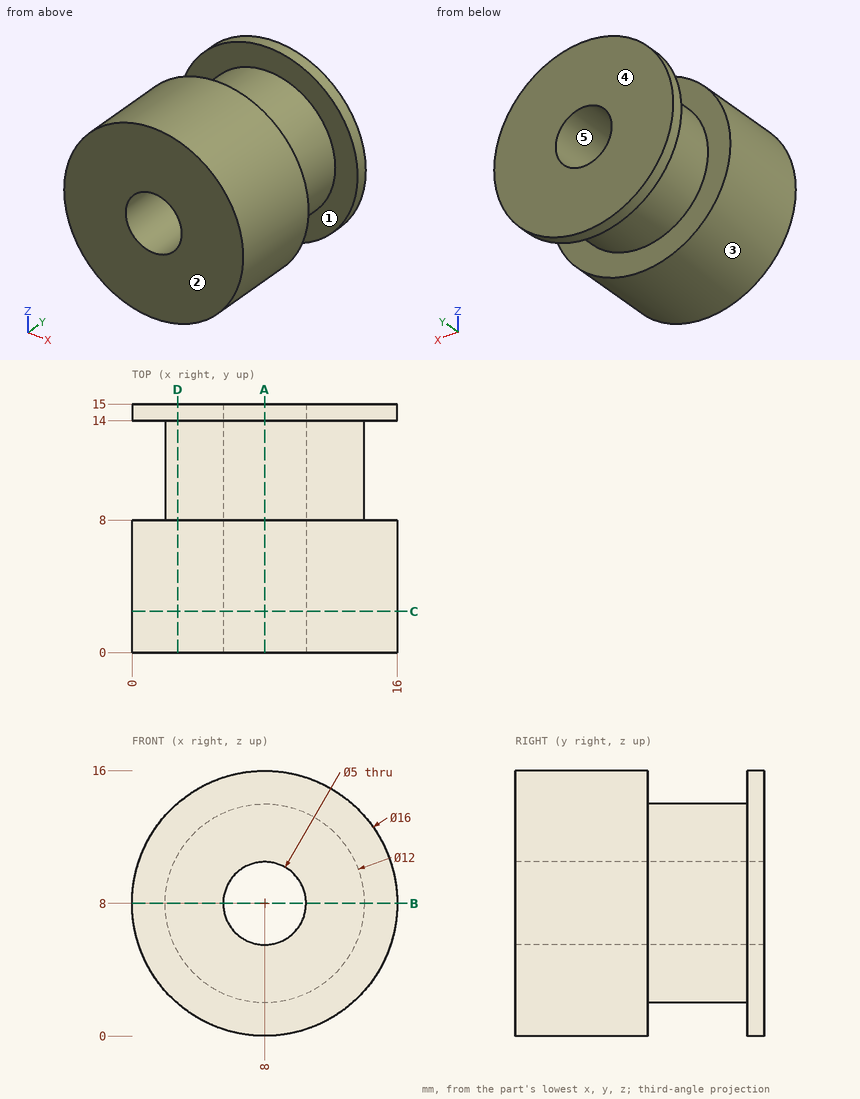
Verification items for this drawing (mm, ordinates from the low corner). A direction names the side the tool comes from. Coordinates: 2 decimals unless noted, no trailing zeros. Loops run counter-clockwise (first coordinate to the right, second up) from the corner with the lowest first, then second, coordinate; pieces in that order, holes last. Notation, with made-up numbers: (-39, 33.5) - (-17, 33.5) arc R15 ccw to (-17, 45.5) - close; hole circle Ø1 at (8, 26). An arc over 180 degrees is marked (long way). One line per item, written item: value. Start each with the question number.
(1) Depth check by flat-ended pin: P1, Ø4, axis at x = 11.5, y = 7, coming from the -Z side; P2, Ø3, axis at y = 5.5, z = 10.5, coming from the -X side; P3, Ø2, axis at x = 5.5, y = 9.5, coming from the +Z side. Enter the tip coordinate at first touch or a pass-through.
(2) Cross-section at A-A on x = 8. Enter the section's corners in (y, z).
(3) Mould release check, pull along X, two halves, no side actions. Record for the marked faces 3, 4 and 5: released by +X, released by -X, zero draft, split by the parting line, or undercut.
(4) Cross-section at C-C on y = 2.5. Enter the section's corners in (x, z), plus the area to 3 significant figures.
(5) Cross-section at B-B on z = 8. Enter the section's corners in (x, y), plus the area to 3 significant figures.
(6) Cross-section at D-D on x = 2.75. Enter the section's corners in (y, z), plus the area to 3 significant figures.
(7) Material ranges on line 1 (Z direction, x = 8, y = 7.25); line 2 (Z direction, x = 8, y = 8.5), recorded low to high. Write a range as [from, to].
(8) Tool access check on the marked faces 1 and 2. Record the directions out of +Z, -Z, +X, -X, +Y, -Y that give a thin tool (end or side, any length) a straight path to the whole face; none if there is none.
Results below:
1. P1: stops at z = 0.14
1. P2: stops at x = 0.06
1. P3: stops at z = 13.81
2. outline: (0, 0) - (8, 0) - (8, 2) - (14, 2) - (14, 0) - (15, 0) - (15, 5.5) - (0, 5.5) - close; (0, 10.5) - (15, 10.5) - (15, 16) - (14, 16) - (14, 14) - (8, 14) - (8, 16) - (0, 16) - close
3. face 3: split by the parting line
3. face 4: zero draft
3. face 5: undercut
4. outline: circle Ø16 at (8, 8); hole circle Ø5 at (8, 8)
4. area: 181 mm2
5. outline: (0, 0) - (5.5, 0) - (5.5, 15) - (0, 15) - (0, 14) - (2, 14) - (2, 8) - (0, 8) - close; (10.5, 0) - (16, 0) - (16, 8) - (14, 8) - (14, 14) - (16, 14) - (16, 15) - (10.5, 15) - close
5. area: 141 mm2
6. outline: (0, 1.96) - (8, 1.96) - (8, 5.1) - (14, 5.1) - (14, 1.96) - (15, 1.96) - (15, 14.04) - (14, 14.04) - (14, 10.9) - (8, 10.9) - (8, 14.04) - (0, 14.04) - close
6. area: 144 mm2
7. line 1: z = [0, 5.5], [10.5, 16]
7. line 2: z = [2, 5.5], [10.5, 14]
8. face 1: none
8. face 2: +Z, -Z, +X, -X, -Y
